The listing builds one solid part. Answer for the finished solid, in the listing's coordinates (mm). Give positions to 0.01 mm unless a question says otherwise; leave off trailing zeros. Order: outer loops, then holes, each group sorted by start corner. A loop starts at its lowest first (then second) coordinate and runs counter-clockwise, first axis right, second up. Notation, with made-up numbers: (22.25, -40) - (59.25, -40) arc R21 ccw to (59.25, -18) - close; hole circle Ø3 at (62.5, 45). An arc over 180 degrees is marked (long way). Answer in a Markdown table with one row per item. Add a question column.
```python
from build123d import *

# Parameters (mm, degrees)
BOSS_EXTRUDE1_DEPTH     = 20
FILLET1_R               = 10
TAP_DRILL_FOR_M5_TAP1_D = 4.2
M5_CLEARANCE_HOLE1_D    = 5.5
TAP_DRILL_FOR_M5_TAP2_D = 4.2
FILLET2_R               = 4


with BuildPart() as part:
    # Sketch1 → Boss-Extrude1 (new body)
    with BuildSketch(Plane.XY):
        with BuildLine():
            Line((-170.200000001, 540.824594888), (-129.309401077, 470))
            Line((-129.309401077, 470), (-93, 470))
            ThreePointArc((-93, 470), (-90.878679656, 470.878679656), (-90, 473))
            Line((-90, 473), (-90, 564.25527297))
            Line((-90, 564.25527297), (-116.225329238, 607))
            Line((-116.225329238, 607), (-170.200000001, 607))
            Line((-170.200000001, 607), (-170.200000001, 540.824594888))
        make_face()
    extrude(amount=BOSS_EXTRUDE1_DEPTH)

    # Fillet1
    fillet1_edges = [part.edges().sort_by_distance(p)[0] for p in [
        (-90, 564.25527297, 10),
        (-129.309401077, 470, 10),
        (-170.200000001, 540.824594888, 10),
    ]]
    fillet(fillet1_edges, radius=FILLET1_R)

    # Tap Drill for M5 Tap1 (through all)
    with Locations(Plane(origin=(0, 0, 0), x_dir=(-1, 0, 0), z_dir=(0, 0, -1))):
        with Locations((119.000000001, 595), (119.000000001, 577), (165.000000001, 577), (165.000000001, 595)):
            Hole(TAP_DRILL_FOR_M5_TAP1_D / 2)

    # M5 Clearance Hole1 (through all)
    with Locations(Plane.XY.offset(20)):
        with Locations((-95, 545), (-125, 545), (-125, 475), (-95, 475), (-110, 490), (-110, 530)):
            Hole(M5_CLEARANCE_HOLE1_D / 2)

    # Tap Drill for M5 Tap2 (through all)
    with Locations(Plane.XY.offset(20)):
        with Locations((-165.570000001, 553.43), (-165.570000001, 600.57), (-118.430000001, 553.43), (-118.430000001, 600.57)):
            Hole(TAP_DRILL_FOR_M5_TAP2_D / 2)

    # Fillet2
    fillet2_edges = [part.edges().sort_by_distance(p)[0] for p in [
        (-116.225329238, 607, 10),
        (-170.200000001, 607, 10),
    ]]
    fillet(fillet2_edges, radius=FILLET2_R)


solid = part.part
```
(1) Straight lines are drawn through the part: line 1 (X direction, y = 545, z = 10); line 2 (Y direction, x = -117.5, z = 18.5); line 3 (Y direction, x = -126.5, z = 13). For each, find the intervals that lie inside material, in ascending order.
(2) Find section D-D, the plane y = 490. Write down the section's boundary in (x, z), plus the area to 3 significant figures.
(3) Find section C-C, the plane x = -110. Write down the section's boundary in (y, z).
(4) The mould has two halves that part along Y. Classify faces 1 (the face through (-109.642, 532.727, 9.86)), 2 (the face through (-128.599, 471.377, 10.14)), 3 (the face through (-119.399, 598.707, 9.86)), 4 (the face through (-170.2, 574, 10)): +Y half, -Y half, draft (parallel to the pull), parting line (faces both ways), or undercut.
(5) Find section B-B, the plane z = 17.5. Give the number of separate pieces and of enclosed holes in the cut face, plus the area to 3 significant figures.
(6) Each of these flat-tipped pins is pushed along its axis until it touches: P1, Ø5.5, axis at x = -118.43, y = 600.57, coming from the -Z side; P2, Ø3.5, axis at x = -165.57, y = 600.57, coming from the +Z side; P3, Ø3, axis at x = -125.5, z = 7, coming from the -Y side. Where does it stop, or does it pass through?
(7) Find section A-A, the plane y = 553.43. Write down the section's boundary in (x, z).
Answer key:
| question | item | result |
|---|---|---|
| 1 | line 1 | -170.2 to -127.75, -122.25 to -97.75, -92.25 to -90 |
| 1 | line 2 | 470 to 551.55, 555.31 to 575.53, 578.47 to 593.53, 596.47 to 598.69, 602.45 to 606.88 |
| 1 | line 3 | 470.45 to 472.7, 477.3 to 542.7, 547.3 to 607 |
| 2 | outline | (-140.86, 0) - (-112.75, 0) - (-112.75, 20) - (-140.86, 20) - close; (-107.25, 0) - (-90, 0) - (-90, 20) - (-107.25, 20) - close |
| 2 | area | 907 mm² |
| 3 | outline | (470, 0) - (487.25, 0) - (487.25, 20) - (470, 20) - close; (492.75, 0) - (527.25, 0) - (527.25, 20) - (492.75, 20) - close; (532.75, 0) - (596.85, 0) - (596.85, 20) - (532.75, 20) - close |
| 4 | face 1 | undercut |
| 4 | face 2 | -Y half |
| 4 | face 3 | undercut |
| 4 | face 4 | draft |
| 5 | separate pieces | 1 |
| 5 | enclosed holes | 14 |
| 5 | area | 8,710 mm² |
| 6 | P1 | z = 0 |
| 6 | P2 | through |
| 6 | P3 | y = 470.01 |
| 7 | outline | (-170.2, 0) - (-167.67, 0) - (-167.67, 20) - (-170.2, 20) - close; (-163.47, 0) - (-120.53, 0) - (-120.53, 20) - (-163.47, 20) - close; (-116.33, 0) - (-90, 0) - (-90, 20) - (-116.33, 20) - close |
